```python
from build123d import *

# Parameters (mm, degrees)
CROQUIS1_W              = 40
CROQUIS1_H              = 60
SALIENTE_EXTRUIR1_DEPTH = 250
CROQUIS2_W              = 34
CROQUIS2_H              = 60
CORTAR_EXTRUIR1_DEPTH   = 50
CROQUIS3_R              = 5
CORTAR_EXTRUIR2_DEPTH   = 255.95097568
CORTAR_EXTRUIR5_DEPTH   = 255.95097568
CROQUIS6_R              = 50
SALIENTE_EXTRUIR2_DEPTH = 5
CROQUIS7_W              = 34
CROQUIS7_H              = 36.99441271
CORTAR_EXTRUIR6_DEPTH   = 221.794021658


with BuildPart() as part:
    # Croquis1 → Saliente-Extruir1 (new body)
    with BuildSketch(Plane(origin=(0, 0, 0), x_dir=(1, 0, 0), z_dir=(0, 1, 0))):
        Rectangle(CROQUIS1_W, CROQUIS1_H)
    extrude(amount=SALIENTE_EXTRUIR1_DEPTH)

    # Croquis2 → Cortar-Extruir1 (cut)
    with BuildSketch(Plane(origin=(0, 250, 0), x_dir=(1, 0, 0), z_dir=(0, 1, 0))):
        Rectangle(CROQUIS2_W, CROQUIS2_H)
    extrude(amount=-CORTAR_EXTRUIR1_DEPTH, mode=Mode.SUBTRACT)

    # Croquis3 → Cortar-Extruir2 (cut, through all)
    with BuildSketch(Plane(origin=(20, 0, 0), x_dir=(0, 0, -1), z_dir=(1, 0, 0))):
        with Locations((-15, 225)):
            Circle(CROQUIS3_R)
    extrude(amount=-CORTAR_EXTRUIR2_DEPTH, mode=Mode.SUBTRACT)

    # Croquis5 → Cortar-Extruir5 (cut, through all)
    with BuildSketch(Plane(origin=(20, 0, 0), x_dir=(0, 0, -1), z_dir=(1, 0, 0))):
        with BuildLine():
            Line((9.840871205, 227.816224024), (30, 50))
            Line((30, 50), (30, 250))
            Line((30, 250), (-15.00000011, 250))
            ThreePointArc((-15.00000011, 250), (1.652243042, 243.646790653), (9.840871205, 227.816224024))
        make_face()
        with BuildLine():
            ThreePointArc((-30, 245), (-22.905694203, 248.717082434), (-15.00000011, 250))
            Line((-15.00000011, 250), (-30, 250))
            Line((-30, 250), (-30, 245))
        make_face()
    extrude(amount=-CORTAR_EXTRUIR5_DEPTH, mode=Mode.SUBTRACT)

    # Croquis6 → Saliente-Extruir2 (add)
    with BuildSketch(Plane.XZ):
        with Locations(Location((0, 15, 0), (0, 0, 270))):
            Circle(CROQUIS6_R)
    extrude(amount=SALIENTE_EXTRUIR2_DEPTH)

    # Croquis7 → Cortar-Extruir6 (cut, through all)
    with BuildSketch(Plane(origin=(0, 200, 0), x_dir=(1, 0, 0), z_dir=(0, 1, 0))):
        with Locations((0, -8.502793645)):
            Rectangle(CROQUIS7_W, CROQUIS7_H)
    extrude(amount=-CORTAR_EXTRUIR6_DEPTH, mode=Mode.SUBTRACT)


solid = part.part
```
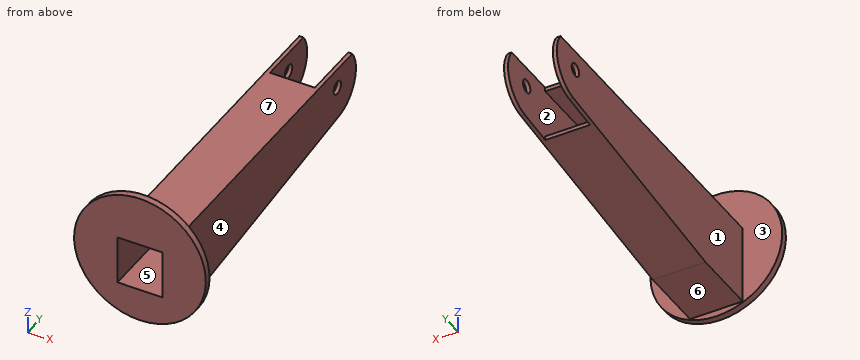
Part model, mm, in its own coordinate system. Face numbers are marked on the shaded views. A direction names the side the tool comes from. Round coordinates to 2 decimals unless told otherwise and drop trailing zeros. Write each loop counter-clockwise with the first axis right and the second up, starting at its lowest first coordinate (ties: lowest second). Pieces come first, ordered by that corner, then holes. Notation, with made-up numbers: (-1, -30.5) -> (50, -30.5) arc R11 ccw to (50, -19.5) -> close; hole circle Ø5 at (60.5, -13.5). An arc over 180 degrees is marked (long way). Return JSON: item names as keys, results as strings. Group by question number.
Q1. Saw through at D-D on y = 225. Write the cut outline in (x, z).
Q2. Pin check, flat tips, straight feed: pin 1 (20 mm diameter, centred on x = 2.5, y = 140.5, fed in from +Z); pin 2 (13 mm diameter, centred on y = 143, z = 2, fed in from +X); pin 3 (13 mm diameter, centred on y = 225, z = 15, fed in from -X). Stop position of each tip, or through.
Q3. Saw through at B-B on y = 16. Write the cut outline in (x, z).
Q4. Mould opens along X. For the marked faces 1, 2, 3 and 4 say: pulls with the +X half, pulls with the -X half, needs draft (parallel to the pull), parting line crosses it, or undercut.
Q5. Saw through at A-A on x = 0. Write the cut outline in (y, z).
Q6. Saw through at C-C on z = 7.5. Write the cut outline in (x, y).
Q7. Probe L1, parallel to X at y = 11.5, z = -2.5; L2, parallel to Y at x = -42, z = 41.5; L3, parallel to X at y = 31, z = -29. List the from-to ranges inside material, lowest first. Write a range as [from, to].
Q8. Which spindle directions (+Z, -Z, +X, -X, +Y, -Y) get a long thin tool onto all of the face, cutting with end or side? Do the marked faces 5, 6 and 7. Say none if no direction does.
Answer:
{
 "1": {"outline": "(-20, -10.16) -> (-17, -10.16) -> (-17, 10) -> (-20, 10) -> close; (-20, 20) -> (-17, 20) -> (-17, 30) -> (-20, 30) -> close; (17, -10.16) -> (20, -10.16) -> (20, 10) -> (17, 10) -> close; (17, 20) -> (20, 20) -> (20, 30) -> (17, 30) -> close"},
 "2": {"pin 1": "z = 30", "pin 2": "x = 20", "pin 3": "x = -20"},
 "3": {"outline": "(-20, -30) -> (20, -30) -> (20, 30) -> (-20, 30) -> close; hole (-17, -9.99) -> (17, -9.99) -> (17, 27) -> (-17, 27) -> close"},
 "4": {"face 1": "pulls with the -X half", "face 2": "undercut", "face 3": "needs draft", "face 4": "pulls with the +X half"},
 "5": {"outline": "(-5, -35) -> (0, -35) -> (0, -30) -> (50, -30) -> (200, -12.99) -> (200, -9.99) -> (-5, -9.99) -> close; (-5, 27) -> (200, 27) -> (200, 30) -> (0, 30) -> (0, 65) -> (-5, 65) -> close"},
 "6": {"outline": "(-49.43, -5) -> (-17, -5) -> (-17, 248.85) -> (-20, 248.85) -> (-20, 0) -> (-49.43, 0) -> close; (17, -5) -> (49.43, -5) -> (49.43, 0) -> (20, 0) -> (20, 248.85) -> (17, 248.85) -> close"},
 "7": {"L1": "[-20, -17], [17, 20]", "L2": "[-5, 0]", "L3": "[-20, 20]"},
 "8": {"face 5": "+Y, -Y", "face 6": "-Z, +X, -X, +Y", "face 7": "+Z, +X, -X, +Y"}
}
